from build123d import *

# Parameters (mm, degrees)
SKETCH1_W                      = 21
SKETCH1_H                      = 25
BOSS_EXTRUDE1_DEPTH            = 4
F_3_1_3_1_DIAMETER_HOLE1_D     = 3.1
F_3_1_3_1_DIAMETER_HOLE1_DEPTH = 10
F_3_1_3_1_DIAMETER_HOLE1_TIP   = 0.931333959
M4X0_7_TAPPED_HOLE1_D          = 3.3


with BuildPart() as part:
    # Sketch1 → Boss-Extrude1 (new body)
    with BuildSketch(Plane(origin=(0, 0, 0), x_dir=(1, 0, 0), z_dir=(0, 1, 0))):
        with Locations((10.5, 12.5)):
            Rectangle(SKETCH1_W, SKETCH1_H)
    extrude(amount=BOSS_EXTRUDE1_DEPTH)

    # Ø3.1 (3.1) Diameter Hole1
    with Locations(Plane(origin=(0, 4, 0), x_dir=(1, 0, 0), z_dir=(0, 1, 0))):
        with Locations((3, 5), (18, 5)):
            Hole(F_3_1_3_1_DIAMETER_HOLE1_D / 2, depth=F_3_1_3_1_DIAMETER_HOLE1_DEPTH)
            with Locations((0, 0, -(F_3_1_3_1_DIAMETER_HOLE1_DEPTH + F_3_1_3_1_DIAMETER_HOLE1_TIP / 2))):  # 118° drill point
                Cone(0, F_3_1_3_1_DIAMETER_HOLE1_D / 2, F_3_1_3_1_DIAMETER_HOLE1_TIP, mode=Mode.SUBTRACT)

    # M4x0.7 Tapped Hole1 (through all)
    with Locations(Plane(origin=(0, 4, 0), x_dir=(1, 0, 0), z_dir=(0, 1, 0))):
        with Locations((10.5, 10), (10.5, 20), (10.5, 15)):
            Hole(M4X0_7_TAPPED_HOLE1_D / 2)


solid = part.part
Input: part model. Units: mm. Frame: model coordinates. Give positions to 0.01 mm unless a question says otherwise; leave off trailing zeros. Write each loop counter-clockwise with the first axis right and the second up, starting at its lowest first coordinate (ties: lowest second). Pieces come first, ordered by that corner, then holes. Notation, with made-up numbers: M 32.5,12 L 72.5,12 A21 cw 72.5,46 Z; hole C 38.5,48 d3. An arc over 180 degrees is marked long. Write item = value, one per line. Start each with the question number.
1) Cut plane B-B on z = -5. Return the cut outline in (x, y).
2) Material intervals for line 1 along Z through (x, y) = (10.5, 3.1); line 2 along X through (y, z) = (0.7, -3.75); line 3 along X through (y, z) = (2.1, -20), sorted ascending. Write a range as [from, to].
3) Cut plane A-A on x = 10.5. Return the cut outline in (y, z), then the cut area to 3 significant figures.
4) Cut plane C-C on x = 18. Return the cut outline in (y, z).
5) Draft query along X for faces 1 (the flat face through (0, 2, -12)), 2 (the cylindrical face through (16.568, 1.972, -4.406)), 3 (the flat face through (10, 2, 0)), 4 (the flat face through (21, 2, -12)). Return one class per face: +X half, -X half, draft (parallel to the pull), parting line (faces both ways), or undercut.
6) Cut plane D-D on z = -20. Return the cut outline in (x, y), then the cut area to 3 significant figures.
7) First-contact query: pin 1 Ø2 at (x, y) = (10, 1) entering from +Z. Flat tip, straight axial feed; report the tip coordinate or a pass-through.
Solved:
q1.outline = M 0,0 L 1.45,0 L 1.45,4 L 0,4 Z; M 4.55,0 L 16.45,0 L 16.45,4 L 4.55,4 Z; M 19.55,0 L 21,0 L 21,4 L 19.55,4 Z
q2.line_1 = [-25, -21.65], [-18.35, -16.65], [-13.35, -11.65], [-8.35, 0]
q2.line_2 = [0, 2.08], [3.92, 17.08], [18.92, 21]
q2.line_3 = [0, 8.85], [12.15, 21]
q3.outline = M 0,-25 L 4,-25 L 4,-21.65 L 0,-21.65 Z; M 0,-18.35 L 4,-18.35 L 4,-16.65 L 0,-16.65 Z; M 0,-13.35 L 4,-13.35 L 4,-11.65 L 0,-11.65 Z; M 0,-8.35 L 4,-8.35 L 4,0 L 0,0 Z
q3.area = 60.4 mm2
q4.outline = M 0,-25 L 4,-25 L 4,-6.55 L 0,-6.55 Z; M 0,-3.45 L 4,-3.45 L 4,0 L 0,0 Z
q5.face_1 = -X half
q5.face_2 = undercut
q5.face_3 = draft
q5.face_4 = +X half
q6.outline = M 0,0 L 8.85,0 L 8.85,4 L 0,4 Z; M 12.15,0 L 21,0 L 21,4 L 12.15,4 Z
q6.area = 70.8 mm2
q7.pin_1 = 0
